from build123d import *

# Parameters (mm, degrees)
ESQUISSE1_W                     = 85
ESQUISSE1_H                     = 70
BOSS_EXTRU_1_DEPTH              = 6
ESQUISSE3_R                     = 1.5
ENL_V_MAT_EXTRU_5_DEPTH         = 5
ESQUISSE5_R                     = 1.75
ENL_V_MAT_EXTRU_6_DEPTH         = 6
R_P_TITION_LIN_AIRE2_COUNT      = 6
R_P_TITION_LIN_AIRE2_PITCH      = 12
R_P_TITION_LIN_AIRE2_COUNT_DIR2 = 5
R_P_TITION_LIN_AIRE2_PITCH_DIR2 = 12
ESQUISSE8_R                     = 1.5
ENL_V_MAT_EXTRU_8_DEPTH         = 5


with BuildPart() as part:
    # Esquisse1 → Boss.-Extru.1 (new body)
    with BuildSketch(Plane.XY):
        Rectangle(ESQUISSE1_W, ESQUISSE1_H)
    extrude(amount=BOSS_EXTRU_1_DEPTH)

    # Esquisse3 → Enlèv. mat.-Extru.5 (cut)
    with BuildSketch(Plane.ZY.offset(42.5)):
        with Locations((3, 0)):
            Circle(ESQUISSE3_R)
    enl_v_mat_extru_5 = extrude(amount=-ENL_V_MAT_EXTRU_5_DEPTH, mode=Mode.SUBTRACT)

    # Symétrie1: Enlèv. mat.-Extru.5 across plane
    add(enl_v_mat_extru_5.mirror(Plane(origin=(0, 0, 0), x_dir=(0, 0, 1), z_dir=(1, 0, 0))), mode=Mode.SUBTRACT)

    # Esquisse5 → Enlèv. mat.-Extru.6 (cut)
    with BuildSketch(Plane.XY):
        with Locations(Location((-31.5, -24, 0), (0, 0, 180))):
            Circle(ESQUISSE5_R)
    enl_v_mat_extru_6 = extrude(amount=ENL_V_MAT_EXTRU_6_DEPTH, mode=Mode.SUBTRACT)

    # Répétition linéaire2: Enl_v. mat.-Extru.6 6 × 5
    with Locations(*[(i * R_P_TITION_LIN_AIRE2_PITCH, j * R_P_TITION_LIN_AIRE2_PITCH_DIR2, 0) for i in range(R_P_TITION_LIN_AIRE2_COUNT) for j in range(R_P_TITION_LIN_AIRE2_COUNT_DIR2) if (i, j) != (0, 0)]):
        add(enl_v_mat_extru_6, mode=Mode.SUBTRACT)

    # Esquisse8 → Enlèv. mat.-Extru.8 (cut)
    with BuildSketch(Plane(origin=(0, 35, 0), x_dir=(1, 0, 0), z_dir=(0, 1, 0))):
        with Locations(Location((0, -3, 0), (0, 0, 270))):
            Circle(ESQUISSE8_R)
    enl_v_mat_extru_8 = extrude(amount=-ENL_V_MAT_EXTRU_8_DEPTH, mode=Mode.SUBTRACT)

    # Symétrie2: Enlèv. mat.-Extru.8 across plane
    add(enl_v_mat_extru_8.mirror(Plane.ZX), mode=Mode.SUBTRACT)


solid = part.part
Model file for the job. Use its own axes, mm. Give positions to 0.01 mm unless a question says otherwise; leave off trailing zeros. Order: outer loops, then holes, each group sorted by start corner. A loop starts at its lowest first (then second) coordinate and runs counter-clockwise, first axis right, second up. Notation, with made-up numbers: (63, 20.25) - (110, 20.25) arc R29 ccw to (110, 40.25) - close; hole circle Ø5 at (48.25, 50.25). An arc over 180 degrees is marked (long way). Write item = value, one per line. Start each with the question number.
1. Cut at A-A, the plane y = 12. List the corners of the cut face in (x, z), and give its area (3 significant figures).
2. Drop flat-ended pins along their axis: P1, Ø2.5, axis at y = 0, z = 3, coming from the +X side; P2, Ø1.5, axis at y = 0, z = 3, coming from the -X side; P3, Ø3, axis at x = 16.5, y = -12, coming from the +Z side; P4, Ø2.5, axis at x = 0, z = 3, coming from the +Y side. Give the stop position or say it passes through.
3. Probe line 1 along Y through (x, z) = (16.5, 2); line 2 along Y through (x, z) = (5.5, 2.4). List the from-to ranges inside material, lowest first.
4. Cut at C-C, the plane x = 29. List the corners of the cut face in (y, z).
5. Cut at D-D, the plane z = 2.7. State how many separate pieces and enclosed holes the cut face has, and give its area (3 significant figures).
6. Cut at B-B, the plane x = -7.5. List the corners of the cut face in (y, z), and give its area (3 significant figures).
7. Two-plate mould, pull along X, no slides. Class faces 1 (the flat face through (-1, 0, 6)), 2 (the flat face through (-37.5, 0, 3)), 3 (the cylindrical face through (-29.75, 11.92, 2.96)), 4 (the cylindrical face through (-30.21, -25.18, 2.96)): pulls with the +X half, pulls with the -X half, needs draft (parallel to the pull), parting line crosses it, or undercut.
Taken from the geometry:
q1.outline = (-42.5, 0) - (-33.25, 0) - (-33.25, 6) - (-42.5, 6) - close; (-29.75, 0) - (-21.25, 0) - (-21.25, 6) - (-29.75, 6) - close; (-17.75, 0) - (-9.25, 0) - (-9.25, 6) - (-17.75, 6) - close; (-5.75, 0) - (2.75, 0) - (2.75, 6) - (-5.75, 6) - close; (6.25, 0) - (14.75, 0) - (14.75, 6) - (6.25, 6) - close; (18.25, 0) - (26.75, 0) - (26.75, 6) - (18.25, 6) - close; (30.25, 0) - (42.5, 0) - (42.5, 6) - (30.25, 6) - close
q1.area = 384 mm²
q2.P1 = 37.5
q2.P2 = -37.5
q2.P3 = through
q2.P4 = 30
q3.line_1 = -35 to -25.75, -22.25 to -13.75, -10.25 to -1.75, 1.75 to 10.25, 13.75 to 22.25, 25.75 to 35
q3.line_2 = -35 to -25.44, -22.56 to -13.44, -10.56 to -1.44, 1.44 to 10.56, 13.44 to 22.56, 25.44 to 35
q4.outline = (-35, 0) - (-25.68, 0) - (-25.68, 6) - (-35, 6) - close; (-22.32, 0) - (-13.68, 0) - (-13.68, 6) - (-22.32, 6) - close; (-10.32, 0) - (-1.68, 0) - (-1.68, 6) - (-10.32, 6) - close; (1.68, 0) - (10.32, 0) - (10.32, 6) - (1.68, 6) - close; (13.68, 0) - (22.32, 0) - (22.32, 6) - (13.68, 6) - close; (25.68, 0) - (35, 0) - (35, 6) - (25.68, 6) - close
q5.separate_pieces = 1
q5.enclosed_holes = 30
q5.area = 5,600 mm²
q6.outline = (-35, 0) - (-25.75, 0) - (-25.75, 6) - (-35, 6) - close; (-22.25, 0) - (-13.75, 0) - (-13.75, 6) - (-22.25, 6) - close; (-10.25, 0) - (-1.75, 0) - (-1.75, 6) - (-10.25, 6) - close; (1.75, 0) - (10.25, 0) - (10.25, 6) - (1.75, 6) - close; (13.75, 0) - (22.25, 0) - (22.25, 6) - (13.75, 6) - close; (25.75, 0) - (35, 0) - (35, 6) - (25.75, 6) - close
q6.area = 315 mm²
q7.face_1 = needs draft
q7.face_2 = pulls with the -X half
q7.face_3 = undercut
q7.face_4 = undercut
